```python
from build123d import *

# Parameters (mm, degrees)
SKETCH1_R           = 1.6999999999999986
SKETCH1_R_2         = 1.7
BOSS_EXTRUDE1_DEPTH = 2
BOSS_EXTRUDE2_DEPTH = 2
SKETCH3_R           = 6.000000000000001
SKETCH3_R_2         = 1.7
BOSS_EXTRUDE3_DEPTH = 2
FILLET1_R           = 10
FILLET2_R           = 10


with BuildPart() as part:
    # Sketch1 → Boss-Extrude1 (new body)
    with BuildSketch(Plane(origin=(0, 0, 0), x_dir=(1, 0, 0), z_dir=(0, 1, 0))):
        with BuildLine():
            Line((-2.999999999999997, -5.196152422706636), (-2.9999999999999973, -18.20384757729328))
            ThreePointArc((-2.9999999999999045, -18.203847577293313), (-2.417e-14, -29.400000000000006), (2.9999999999999534, -18.20384757729334))
            Line((3.0000000000000027, -18.20384757729332), (3.000000000000003, -5.196152422706632))
            ThreePointArc((3.0000000000000027, -5.196152422706631), (-3.11e-15, 6), (-2.9999999999999973, -5.196152422706634))
        make_face()
        with Locations(Location((-5e-16, -23.400000000000002, 0), (0, 0, 270))):
            Circle(SKETCH1_R, mode=Mode.SUBTRACT)
        with Locations(Location((0, 0, 0), (0, 0, 270))):
            Circle(SKETCH1_R_2, mode=Mode.SUBTRACT)
    boss_extrude1 = extrude(amount=BOSS_EXTRUDE1_DEPTH)

    # Sketch2 → Boss-Extrude2 (add)
    with BuildSketch(Plane(origin=(0, 2, 0), x_dir=(1, 0, 0), z_dir=(0, 1, 0))):
        Polygon((-2.999999999999997, -26.000000000000004), (-2.9999999999999964, -5.196152422706635), (-0.9999999999999996, -5.196152422706635), (-0.999999999999997, -26.000000000000004), align=None)
        Polygon((3.000000000000003, -26.000000000000004), (1.000000000000003, -26.000000000000004), (1.000000000000003, -5.196152422706631), (3.0000000000000027, -5.196152422706631), align=None)
    boss_extrude2 = extrude(amount=BOSS_EXTRUDE2_DEPTH)

    # Sketch3 → Boss-Extrude3 (add)
    with BuildSketch(Plane(origin=(0, 2, 0), x_dir=(1, 0, 0), z_dir=(0, 1, 0))):
        Circle(SKETCH3_R)
        with Locations(Location((0, 0, 0), (0, 0, 270))):
            Circle(SKETCH3_R_2, mode=Mode.SUBTRACT)
    extrude(amount=BOSS_EXTRUDE3_DEPTH)

    # Fillet1
    fillet1_edges = [part.edges().sort_by_distance(p)[0] for p in [
        (-2.999999999999997, 2, 5.196152422706636),
        (3.0000000000000027, 2, 5.196152422706631),
    ]]
    fillet(fillet1_edges, radius=FILLET1_R)

    # Mirror1: Boss-Extrude1, Boss-Extrude2 across plane
    add(boss_extrude1.mirror(Plane.XY))
    add(boss_extrude2.mirror(Plane.XY))

    # Fillet2
    fillet2_edges = [part.edges().sort_by_distance(p)[0] for p in [
        (3.0000000000000027, 2, -5.196152422706631),
        (-2.999999999999997, 2, -5.196152422706636),
    ]]
    fillet(fillet2_edges, radius=FILLET2_R)


solid = part.part
```
The model under review builds one solid part; all positions refer to its coordinate system, in mm. A direction names the side the tool comes from. Coordinates: 2 decimals unless noted, no trailing zeros. Write each loop counter-clockwise with the first axis right and the second up, starting at its lowest first coordinate (ties: lowest second). Pieces come first, ordered by that corner, then holes. Notation, with made-up numbers: (70, 65.5) - (103, 65.5) arc R20 cw to (103, 85.5) - close; hole circle Ø7 at (-31.5, 6.25). An arc over 180 degrees is marked (long way). Write item = value, one per line.
(1) For P1, Ø1, axis at y = 1.5, z = 2.5, coming from the -X side; P2, Ø1, axis at y = 3.5, z = -16, coming from the -X side; P3, Ø1.5, axis at x = -2.5, y = 3, coming from the +Z side, all flat-tipped, find the tip position at first contact; note any pin that passes through.
Result sheet:
P1 = -5.66
P2 = -3
P3 = 26
(2) Consider section C-C, the plane y = 1.35. Give the boundary of the cut face in (x, z) (3 decimals).
Result sheet:
outline = (-4.875, -3.498) arc R10 cw to (-3, -9.327) - (-3, -18.204) arc R6 ccw (long way) to (3, -18.204) - (3, -9.327) arc R10 cw to (4.875, -3.498) arc R6 ccw to (4.875, 3.498) arc R10 cw to (3, 9.327) - (3, 18.204) arc R6 ccw (long way) to (-3, 18.204) - (-3, 9.327) arc R10 cw to (-4.875, 3.498) arc R6 ccw to start; hole circle Ø3.4 at (0, -23.4); hole circle Ø3.4 at (0, 0); hole circle Ø3.4 at (0, 23.4)
(3) For line 1 (X direction, y = 2.9, z = 19); line 2 (X direction, y = 1.5, z = 23.4); line 3 (X direction, y = 1.9, z = 18), list the stretches that pass through material, from the lowest coordinate up. Write a range as [from, to].
Result sheet:
line_1 = [-3, -1], [1, 3]
line_2 = [-6, -1.7], [1.7, 6]
line_3 = [-3, 3]
(4) Consider section D-D, the plane z = 0. Give the boundary of the cut face in (x, y).
Result sheet:
outline = (-6, 0) - (-1.7, 0) - (-1.7, 4) - (-6, 4) - close; (1.7, 0) - (6, 0) - (6, 4) - (1.7, 4) - close
(5) Mouldability with a two-part tool opening along X and no side actions: class faces 5 (the face through (-3.467, 2.028, -6.307)), 6 (the face through (0, 3, 6)), 7 (the face through (3.5, 2, 6.2)), 8 (the face through (-1, 3, -16)) as pulls with the +X half, pulls with the -X half, needs draft (parallel to the pull), parting line crosses it, or undercut.
Result sheet:
face_5 = pulls with the -X half
face_6 = undercut
face_7 = pulls with the +X half
face_8 = undercut
(6) Machinability: for faces 1 (the face through (-2, 3, 26)), 2 (the face through (3, 2, 16)), 3 (the face through (3.467, 1.972, -6.307)), 4 (the face through (2, 3, -26)), which of the approach directions +Z, -Z, +X, -X, +Y, -Y give a long, thin tool a straight path to every point of the face, cutting with its end or side? Answer none if there is none.
Result sheet:
face_1 = +Z, +X, -X, +Y
face_2 = +X, +Y
face_3 = +X, +Y, -Y
face_4 = -Z, +X, -X, +Y
(7) Consider section B-B, the plane z = 23.4. Give the boundary of the cut face in (x, y), then the cut area to 3 significant figures.
Result sheet:
outline = (-6, 0) - (-1.7, 0) - (-1.7, 2) - (-1, 2) - (-1, 4) - (-3, 4) - (-3, 2) - (-6, 2) - close; (1, 2) - (1.7, 2) - (1.7, 0) - (6, 0) - (6, 2) - (3, 2) - (3, 4) - (1, 4) - close
area = 25.2 mm^2
(8) Consider section A-A, the plane x = 0. Give the boundary of the cut face in (y, z), then the cut area to 3 significant figures.
Result sheet:
outline = (0, -29.4) - (2, -29.4) - (2, -25.1) - (0, -25.1) - close; (0, -21.7) - (2, -21.7) - (2, -6) - (4, -6) - (4, -1.7) - (0, -1.7) - close; (0, 1.7) - (4, 1.7) - (4, 6) - (2, 6) - (2, 21.7) - (0, 21.7) - close; (0, 25.1) - (2, 25.1) - (2, 29.4) - (0, 29.4) - close
area = 114 mm^2
